Autodesk Inventor part; units mm, degrees
ref_plane "YZ Plane" through (0, 0, 0) normal (1, 0, 0) x (0, 1, 0)
ref_plane "XZ Plane" through (0, 0, 0) normal (0, 1, 0) x (-1, 0, 0)
ref_plane "XY Plane" through (0, 0, 0) normal (0, 0, 1) x (1, 0, 0)
sketch "Sketch1" plane through (0, 0, 0) normal (0, 0, 1) x (1, 0, 0)
  line L0 (0, 0) -> (0, 101)
  line L1 (0, 101) -> (10, 101)
  line L2 (10, 101) -> (16, 101)
  line L3 (16, 101) -> (16, 16)
  line L4 (16, 16) -> (101, 16)
  line L5 (101, 16) -> (101, 0)
  line L6 (101, 0) -> (0, 0)
  line L7 (16, 101) -> (13, 101)
  line L8 (13, 101) -> (13, 13)
  line L9 (13, 13) -> (101, 13)
  line L10 (16, 16) -> (13, 16)
  line L11 (16, 16) -> (16, 13)
  line L12 (10, 101) -> (10, 8)
  line L13 (10, 8) -> (101, 8)
  line L14 (16, 13) -> (46, 13)
  line L15 (101, 13) -> (95, 13)
  line L16 (13, 101) -> (13, 95)
  circle A0 centre (95, 13) radius 1.25
  circle A1 centre (46, 13) radius 1.25
  circle A2 centre (13, 95) radius 1.25
  line L17 (13, 16) -> (13, 46)
  circle A3 centre (13, 46) radius 1.25
  line L18 (11.75, 95) -> (11.75, 46)
  line L19 (14.25, 46) -> (14.25, 95)
  line L20 (46, 14.25) -> (95, 14.25)
  line L21 (46, 11.75) -> (95, 11.75)
  point P0 (58.5, 16)
  dimension "d0" = 101
  dimension "d1" = 10
  dimension "d2" = 6
  dimension "d3" = 101
  dimension "d4" = 16
  dimension "d32" = 3
  dimension "d34" = 3
  dimension "d35" = 30
  dimension "d36" = 6
  dimension "d37" = 6
  dimension "d38" = 2.5
  dimension "d39" = 2.5
  dimension "d40" = 2.5
  dimension "d41" = 30
  dimension "d42" = 2.5
extrude "Extrusion1" add sketch "Sketch1" along normal blind 5 contours L0 L1 L12 L13 L5 L6 | L2 L8 A2 L18 A3 L9 A1 L21 A0 L5 L13 L12 | L2 L3 L10 L8 A3 L19 A2 | L9 A0 L20 A1 L11 L4 L5 | L11 L9 L8 L10
sketch "Sketch2" plane through (0, 0, 5) normal (0, 0, 1) x (1, 0, 0)
  line L0 (101, 0) -> (101, 16)
  line L1 (101, 16) -> (16, 16)
  line L2 (16, 16) -> (16, 101)
  line L3 (16, 101) -> (0, 101)
  line L4 (0, 101) -> (0, 0)
  line L5 (0, 0) -> (101, 0)
  line L6 (0, 101) -> (10, 101)
  line L7 (10, 101) -> (10, 10)
  line L8 (10, 10) -> (101, 10)
  line L9 (101, 0) -> (101, 16)
  line L10 (101, 10) -> (101, 0)
  line L11 (101, 0) -> (0, 0)
  line L12 (0, 101) -> (0, 0)
  dimension "d7" = 10
  dimension "d8" = 10
extrude "Extrusion2" add sketch "Sketch2" along normal blind 10 contours L5 L4 L3 L7 L8 L0
sketch "Sketch3" plane through (0, 0, 15) normal (0, 0, 1) x (1, 0, 0)
  line L0 (10, 10) -> (10, 101)
  line L1 (10, 101) -> (0, 101)
  line L2 (0, 101) -> (0, 0)
  line L3 (0, 0) -> (101, 0)
  line L4 (101, 0) -> (101, 10)
  line L5 (101, 10) -> (10, 10)
  line L6 (0, 101) -> (5, 101)
  line L7 (5, 101) -> (5, 5)
  line L8 (5, 5) -> (101, 5)
  line L9 (10, 101) -> (10, 10)
  line L10 (10, 10) -> (101, 10)
  line L11 (101, 10) -> (101, 16)
  line L12 (101, 16) -> (16, 16)
  line L13 (16, 16) -> (16, 101)
  line L14 (16, 101) -> (10, 101)
  line L15 (5, 101) -> (5, 96)
  line L16 (5, 16) -> (5, 21)
  line L17 (16, 5) -> (21, 5)
  line L18 (101, 5) -> (96, 5)
  line L19 (5, 96) -> (5, 71)
  line L20 (5, 71) -> (5, 46)
  line L21 (21, 5) -> (46, 5)
  line L22 (46, 5) -> (71, 5)
  circle A0 centre (5, 96) radius 1.5
  circle A1 centre (5, 71) radius 1.5
  circle A2 centre (5, 46) radius 1.5
  circle A3 centre (5, 21) radius 1.5
  circle A4 centre (21, 5) radius 1.5
  circle A5 centre (46, 5) radius 1.5
  circle A6 centre (71, 5) radius 1.5
  circle A7 centre (96, 5) radius 1.5
  dimension "d11" = 5
  dimension "d12" = 5
  dimension "d13" = 85
  dimension "d14" = 5
  dimension "d15" = 5
  dimension "d16" = 5
  dimension "d17" = 5
  dimension "d18" = 25
  dimension "d19" = 25
  dimension "d20" = 25
  dimension "d21" = 25
  dimension "d22" = 3
  dimension "d23" = 3
  dimension "d24" = 3
  dimension "d25" = 3
  dimension "d26" = 3
  dimension "d27" = 3
  dimension "d28" = 3
  dimension "d29" = 3
  dimension "d47" = 25
  dimension "d48" = 25
extrude "Extrusion3" cut sketch "Sketch3" against normal blind 16 contours A0 L7 | L7 A0 | A7 L8 | L8 A7 | A1 L7 | L7 A1 | A6 L8 | L8 A6 | A2 L7 | L7 A2 | A5 L8 | L8 A5 | A3 L7 | L7 A3 | A4 L8 | L8 A4
fillet "Fillet1" radius 2 11 edges at (5, 101, 15) (10, 101, 10) (16, 101, 2.5) (8, 101, 0) (0, 101, 7.5) (101, 16, 2.5) (101, 8, 0) (101, 13, 5) (101, 10, 10) (101, 5, 15) (101, 0, 7.5)
sketch "Sketch5" plane through (10, 10, 15) normal (1, 0, 0) x (0, 0, -1)
  line L0 (0, 89) -> (10, 89)
  line L1 (0, 0) -> (0, 89)
  line L2 (10, 0) -> (0, 0)
  line L3 (10, 89) -> (10, 0)
  circle A0 centre (26.9628, 94.4324) radius 2
  line L4 (0, 89) -> (10, 89)
  line L5 (10, 89) -> (7.5, 89)
  line L6 (7.5, 89) -> (7.5, 44.5)
  circle A1 centre (7.5, 44.5) radius 2
  point P0 (15, -10)
  dimension "d49" = 10
  dimension "d50" = 89
  dimension "d51" = 4
  dimension "d52" = 2.5
  dimension "d53" = 44.5
  dimension "d54" = 4
extrude "Extrusion4" cut sketch "Sketch5" against normal blind 10 contours A1
sketch "Sketch6" plane through (10, 10, 15) normal (0, 1, 0) x (1, 0, 0)
  line L0 (89, 10) -> (89, 0)
  line L1 (0, 10) -> (89, 10)
  line L2 (0, 10) -> (0, 0)
  line L3 (89, 0) -> (0, 0)
  line L4 (0, 10) -> (0, 7.5)
  line L5 (0, 7.5) -> (44.5, 7.5)
  circle A0 centre (44.5, 7.5) radius 2
  point P0 (-10, 15)
  dimension "d57" = 2.5
  dimension "d58" = 44.5
  dimension "d59" = 4
extrude "Extrusion5" cut sketch "Sketch6" against normal blind 10 contours A0
equation "\"d3\" = d0"
equation "\"d4\" = d1 + d2"
equation "\"d32\" = 0.5 * d2"
equation "\"d36\" = 2 * d32"
equation "\"d37\" = d36"
equation "\"d39\" = d38"
equation "\"d40\" = d38"
equation "\"d41\" = d35"
equation "\"d42\" = d38"
equation "\"d7\" = d1"
equation "\"d8\" = d1"
equation "\"d11\" = 0.5 * d1"
equation "\"d14\" = d11"
equation "\"d15\" = d11"
equation "\"d16\" = d11"
equation "\"d17\" = d11"
equation "\"d18\" = -0.666667 * d14 + 0.333333 * d13"
equation "\"d19\" = d18"
equation "\"d20\" = d18"
equation "\"d21\" = d18"
equation "\"d23\" = d22"
equation "\"d24\" = d22"
equation "\"d25\" = d22"
equation "\"d26\" = d22"
equation "\"d27\" = d22"
equation "\"d28\" = d22"
equation "\"d29\" = d22"
equation "\"d47\" = d18"
equation "\"d48\" = d18"
equation "\"d30\" = d1 + d2"
equation "\"d53\" = 0.5 * d50"
equation "\"d54\" = d51"
equation "\"d57\" = d52"
equation "\"d58\" = d53"
equation "\"d59\" = d54"
properties part number "DUT Holder v1.0"
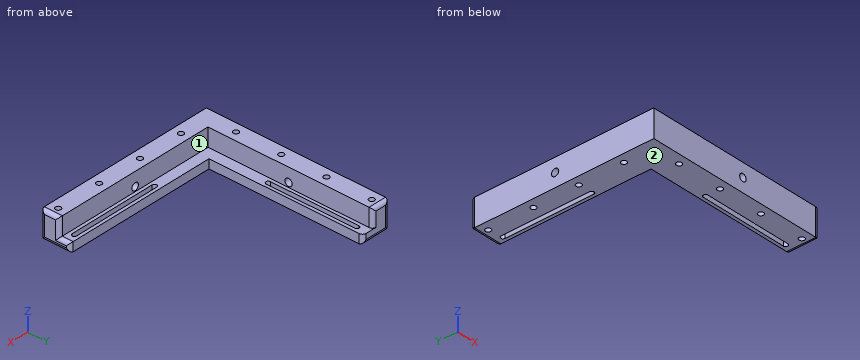
The listing builds one solid part. Answer for the finished solid, in the listing's coordinates (mm). Face numbers are marked on the shaded views. A direction names the side the tool comes from. Give positions to 0.01 mm unless a question says otherwise; leave off trailing zeros. Loops run counter-clockwise (first coordinate to the right, second up) from the corner with the lowest first, then second, coordinate; pieces in that order, holes last. Notation, with made-up numbers: (78.5, -14) - (107.5, -14) arc R30 cw to (107.5, 20) - close; hole circle Ø11 at (-16.5, -28.5). An arc over 180 degrees is marked (long way). Use one line per item in the form item = value.
1. Section C-C on y = 92.5 is taken. Give the vertices of the cut face in (x, z), then the cut area to 4 significant figures.
Calculated:
outline = (0, 0) - (11.75, 0) - (11.75, 5) - (10, 5) - (10, 15) - (0, 15) - close; (14.25, 0) - (16, 0) - (16, 5) - (14.25, 5) - close
area = 167.5 mm^2
2. Find the intervals of material crossed by line 1 along Y through (x, z) = (5, 4); line 2 along Z through (x, y) = (6.5, 54.5), in increasing order. Write a range as [from, to].
Calculated:
line_1 = [0, 19.5], [22.5, 44.5], [47.5, 69.5], [72.5, 94.5], [97.5, 101]
line_2 = [0, 5.5], [9.5, 15]
3. Section A-A on x = 5 is taken. Give the vertices of the cut face in (y, z), then the cut area to 3 significant figures.
Calculated:
outline = (0, 0) - (19.5, 0) - (19.5, 15) - (0, 15) - close; (22.5, 0) - (44.5, 0) - (44.5, 15) - (22.5, 15) - close; (47.5, 0) - (69.5, 0) - (69.5, 15) - (47.5, 15) - close; (72.5, 0) - (94.5, 0) - (94.5, 15) - (72.5, 15) - close; (97.5, 0) - (99, 0) arc R2 ccw to (101, 2) - (101, 13) arc R2 ccw to (99, 15) - (97.5, 15) - close; hole circle Ø4 at (54.5, 7.5)
area = 1,320 mm^2
4. Given pin 1 Ø2.5 at (x, z) = (81.5, 3) entering from +Y; pin 2 Ø1.5 at (y, z) = (15, 3) entering from +X; pin 3 Ø5 at (y, z) = (46, 11) entering from +X, each flat-ended and moving along its own axis, determine where each tip first touches the part or whether it passes through.
Calculated:
pin_1 = 16
pin_2 = 100.98
pin_3 = 10
5. Section D-D on x = 21 is taken. Give the vertices of the cut face in (y, z), then the cut area to 3 significant figures.
Calculated:
outline = (0, 0) - (3.5, 0) - (3.5, 15) - (0, 15) - close; (6.5, 0) - (16, 0) - (16, 5) - (10, 5) - (10, 15) - (6.5, 15) - close
area = 135 mm^2
6. Section B-B on z = 7.5 is taken. Count the separate pieces of the cut face and the enclosed holes in it, then the cut area to 3 significant figures.
Calculated:
separate_pieces = 3
enclosed_holes = 8
area = 1,780 mm^2
7. Which of the six approach directions +Z, -Z, +X, -X, +Y, -Y give full straight-line access (tool end or side, diameter ignored) to the marked faces 1 and 2?
Calculated:
face_1 = +Z, +X, +Y
face_2 = -Z, +X, -X, +Y, -Y
